from build123d import *

# Parameters (mm, degrees)
SKETCH1_R           = 4.3688
SKETCH1_R_2         = 3.048
BOSS_EXTRUDE1_DEPTH = 3.429
BOSS_EXTRUDE2_DEPTH = 2.3114
SKETCH3_R           = 1.5621
CUT_EXTRUDE1_DEPTH  = 21.699383219


with BuildPart() as part:
    # Sketch1 → Boss-Extrude1 (new body)
    with BuildSketch(Plane(origin=(0, 0, 0), x_dir=(1, 0, 0), z_dir=(0, 1, 0))):
        with Locations(Location((0, 0, 0), (0, 0, 270))):
            Circle(SKETCH1_R)
        with Locations(Location((0, 0, 0), (0, 0, 270))):
            Circle(SKETCH1_R_2, mode=Mode.SUBTRACT)
    extrude(amount=BOSS_EXTRUDE1_DEPTH)

    # Sketch2 → Boss-Extrude2 (add)
    with BuildSketch(Plane(origin=(0, 3.429, 0), x_dir=(1, 0, 0), z_dir=(0, 1, 0))):
        with BuildLine():
            Line((5.322708788, 3.823825598), (16.607191493, 2.6416))
            ThreePointArc((16.607191493, 2.6416), (18.9865, 0), (16.607191493, -2.6416))
            Line((16.607191493, -2.6416), (5.322708788, -3.823825598))
            ThreePointArc((5.322708788, -3.823825598), (4.567932808, -4.023552477), (3.909477587, -4.443093093))
            ThreePointArc((3.909477587, -4.443093093), (0, -5.9182), (-3.909477587, -4.443093093))
            ThreePointArc((-3.909477587, -4.443093093), (-4.567932808, -4.023552477), (-5.322708788, -3.823825598))
            Line((-5.322708788, -3.823825598), (-16.607191493, -2.6416))
            ThreePointArc((-16.607191493, -2.6416), (-18.9865, 0), (-16.607191493, 2.6416))
            Line((-16.607191493, 2.6416), (-5.322708788, 3.823825598))
            ThreePointArc((-5.322708788, 3.823825598), (-4.567932808, 4.023552477), (-3.909477587, 4.443093093))
            ThreePointArc((-3.909477587, 4.443093093), (0, 5.9182), (3.909477587, 4.443093093))
            ThreePointArc((3.909477587, 4.443093093), (4.567932808, 4.023552477), (5.322708788, 3.823825598))
        make_face()
    extrude(amount=BOSS_EXTRUDE2_DEPTH)

    # Sketch3 → Cut-Extrude1 (cut, through all)
    with BuildSketch(Plane(origin=(0, 5.7404, 0), x_dir=(1, 0, 0), z_dir=(0, 1, 0))):
        with Locations(Location((0, 0, 0), (0, 0, 270))):
            Circle(SKETCH3_R)
    extrude(amount=-CUT_EXTRUDE1_DEPTH, mode=Mode.SUBTRACT)


solid = part.part
Verification items for the finished model (mm, model axes). A direction names the side the tool comes from. Coordinates: 2 decimals unless noted, no trailing zeros. Order: outer loops, then holes, each group sorted by start corner. A loop starts at its lowest first (then second) coordinate and runs counter-clockwise, first axis right, second up. Notation, with made-up numbers: M -28,-11.5 L -11,-11.5 A22 ccw -11,27.5 Z; hole C 63.25,87.5 d2. An arc over 180 degrees is marked long. One line per item, written item: value. Start each with the question number.
Item 1: Access from +Z, -Z, +X, -X, +Y, -Y to the whole of each face (thin tool, end or side, straight path). Record for faces 1 (the cylindrical face through (18.986, 4.569, -0.055)), 2 (the flat face through (-1.3, 3.429, 1.3)).
Item 2: Sectioned sample at A-A on y = 5.3. Record the cut outline in (x, z).
Item 3: Depth check by flat-ended pin: P1, Ø4, axis at x = 12, z = -4.5, coming from the -Y side; P2, Ø2, axis at x = 13, y = 5, coming from the -Z side; P3, Ø1, axis at x = -12, y = 3.5, coming from the -Z side. Enter the tip coordinate at first touch or a pass-through.
Item 4: Thickness scan on probe 1 along X at (y, z) = (1.2, 0); probe 2 along X at (y, z) = (2, -1.5); probe 3 along Y at (x, z) = (-6.5, 1.75). Record the ranges inside material, lowest first.
Item 5: Sectioned sample at B-B on z = 0.25. Record the cut outline in (x, y), then the cut area to 3 significant figures.
Item 6: Sectioned sample at C-C on x = 0. Record the cut outline in (y, z), then the cut area to 3 significant figures.
Item 7: Mould release check, pull along X, two halves, no side actions. Record for faces 3 (the cylindrical face through (2.57, 1.69, 1.64)), 4 (the cylindrical face through (4.58, 4.57, 4.02)), 5 (the flat face through (-11.044, 4.569, -3.224)): pulls with the +X half, pulls with the -X half, needs draft (parallel to the pull), parting line crosses it, or undercut.
Item 8: Sectioned sample at D-D on y = 2.8. Record the cut outline in (x, z).
Calculated:
1. face 1: +X, +Y, -Y
1. face 2: -Y
2. outline: M -16.61,-2.64 L -5.32,-3.82 A2.54 cw -3.91,-4.44 A5.92 ccw 3.91,-4.44 A2.54 cw 5.32,-3.82 L 16.61,-2.64 A2.66 ccw 16.61,2.64 L 5.32,3.82 A2.54 cw 3.91,4.44 A5.92 ccw -3.91,4.44 A2.54 cw -5.32,3.82 L -16.61,2.64 A2.66 ccw Z; hole C 0,0 d3.12
3. P1: y = 3.43
3. P2: z = -3.12
3. P3: z = -3.18
4. probe 1: -4.37 to -3.05, 3.05 to 4.37
4. probe 2: -4.1 to -2.65, 2.65 to 4.1
4. probe 3: 3.43 to 5.74
5. outline: M -18.97,3.43 L -4.36,3.43 L -4.36,0 L -3.04,0 L -3.04,3.43 L -1.54,3.43 L -1.54,5.74 L -18.97,5.74 Z; M 1.54,3.43 L 3.04,3.43 L 3.04,0 L 4.36,0 L 4.36,3.43 L 18.97,3.43 L 18.97,5.74 L 1.54,5.74 Z
5. area: 89.7 mm^2
6. outline: M 0,-4.37 L 3.43,-4.37 L 3.43,-5.92 L 5.74,-5.92 L 5.74,-1.56 L 3.43,-1.56 L 3.43,-3.05 L 0,-3.05 Z; M 0,3.05 L 3.43,3.05 L 3.43,1.56 L 5.74,1.56 L 5.74,5.92 L 3.43,5.92 L 3.43,4.37 L 0,4.37 Z
6. area: 29.2 mm^2
7. face 3: undercut
7. face 4: pulls with the +X half
7. face 5: pulls with the -X half
8. outline: C 0,0 d8.74; hole C 0,0 d6.1
